Input: part model. Units: mm. Frame: model coordinates. Face numbers are marked on the shaded views. Give positions to 0.01 mm unless a question says otherwise; leave off trailing zeros. Loops run counter-clockwise (first coordinate to the right, second up) from the corner with the lowest first, then second, coordinate; pieces in that order, holes last. Notation, with made-up numbers: M -24,54.5 L 7,54.5 A21 ccw 7,77.5 Z; hole C 39,32 d4. An arc over 180 degrees is marked long. One line per item, written item: value. Start each with the question number.
(1) Pull-direction query (Y, two-part tool) for the marked faces 1, 2 and 3; classes: released by +Y, released by -Y, zero draft, split by the parting line, or undercut.
(2) Section D-D on z = 2.5. Output: boundary loops of the cut face in (x, y), plus the area to 3 significant figures.
(3) Section A-A on x = -0.25. Output: boundary loops of the cut face in (y, z), plus the area to 3 significant figures.
(4) Pin query (flat end, axial travel): P1, Ø1, axis at x = 0.5, z = 3.5, coming from the -Y side; P2, Ø1, axis at x = -0.5, y = 9.5, coming from the -Z side. Return the tip coordinate at first contact, or that it passes through.
(5) Section C-C on x = 0.95. Output: boundary loops of the cut face in (y, z).
(6) Section B-B on y = 1.25. Output: boundary loops of the cut face in (x, z).
(7) Ray query, line 1 along Y through (x, z) = (-0.55, 2.5); line 2 along Y through (x, z) = (-0.85, 4); line 3 along Z through (x, y) = (0.8, 16.5). Return the intervals inside material, ascending. Write a range as from..to.
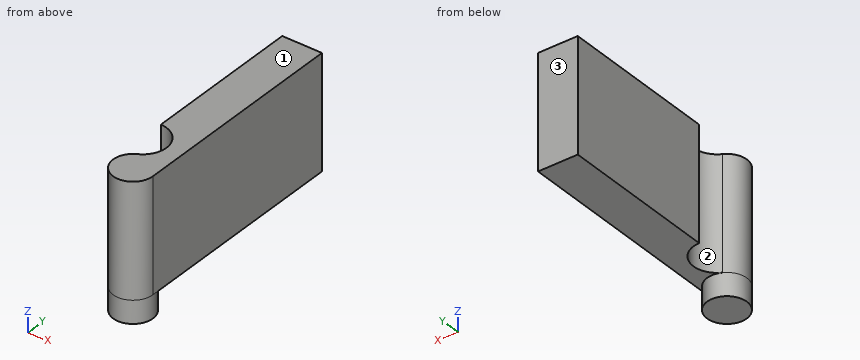
```python
from build123d import *

# Parameters (mm, degrees)
DODANIE_WYCI_GNI_CIE1_DEPTH = 10
SZKIC2_R                    = 1.75
DODANIE_WYCI_GNI_CIE2_DEPTH = 2


with BuildPart() as part:
    # Szkic1 → Dodanie-wyciągnięcie1 (new body)
    with BuildSketch(Plane.XY):
        with BuildLine():
            Line((1.75, 0), (1.75, 19.5))
            Line((1.75, 19.5), (-1.75, 19.5))
            Line((-1.75, 19.5), (-1.75, 5.5))
            ThreePointArc((-1.75, 5.5), (0.277964608, 3.903301802), (-0.798314607, 1.557303371))
            ThreePointArc((-0.798314607, 1.557303371), (-0.912537517, -1.493243209), (1.75, 0))
        make_face()
    extrude(amount=DODANIE_WYCI_GNI_CIE1_DEPTH)

    # Szkic2 → Dodanie-wyciągnięcie2 (add)
    with BuildSketch(Plane(origin=(0, 0, 0), x_dir=(-1, 0, 0), z_dir=(0, 0, -1))):
        Circle(SZKIC2_R)
    extrude(amount=DODANIE_WYCI_GNI_CIE2_DEPTH)


solid = part.part
```
Output values:
1. face 1: zero draft
1. face 2: undercut
1. face 3: released by +Y
2. outline: M -1.75,5.5 A2.09 cw -0.8,1.56 A1.75 ccw long 1.75,0 L 1.75,19.5 L -1.75,19.5 Z
2. area: 65.9 mm²
3. outline: M -1.73,-2 L 1.73,-2 L 1.73,0 L 1.96,0 L 1.96,10 L -1.73,10 Z; M 4.86,0 L 19.5,0 L 19.5,10 L 4.86,10 Z
3. area: 190 mm²
4. P1: stops at y = -1.75
4. P2: stops at z = 0
5. outline: M -1.47,-2 L 1.47,-2 L 1.47,0 L 19.5,0 L 19.5,10 L -1.47,10 Z
6. outline: M -1.22,-2 L 1.22,-2 L 1.22,0 L 1.75,0 L 1.75,10 L -1.22,10 Z
7. line 1: y = -1.66..1.71, 5.12..19.5
7. line 2: y = -1.53..1.53, 5.3..19.5
7. line 3: z = 0..10
